Autodesk Inventor part; units mm, degrees
ref_plane "YZ Plane" through (0, 0, 0) normal (1, 0, 0) x (0, 1, 0)
ref_plane "XZ Plane" through (0, 0, 0) normal (0, 1, 0) x (-1, 0, 0)
ref_plane "XY Plane" through (0, 0, 0) normal (0, 0, 1) x (1, 0, 0)
sketch "Эскиз1" plane through (0, 0, 0) normal (0, 1, 0) x (-1, 0, 0)
  arc A0 (-8.6049, 20.7741) -> (-8.0517, 15.4673) centre (8.9595, 19.9228) ccw
  arc A1 (-8.0517, 15.4673) -> (-9.3692, 14.7066) centre (0, 0) ccw
  arc A2 (-9.3692, 14.7066) -> (-13.6885, 17.8391) centre (-21.7334, 2.2022) ccw
  arc A3 (-13.6885, 17.8391) -> (-15.1912, 16.5782) centre (0, 0) ccw
  arc A4 (-15.1912, 16.5782) -> (-12.8563, 11.7806) centre (1.6052, 21.7856) ccw
  arc A5 (-12.8563, 11.7806) -> (-13.8341, 10.6153) centre (0, 0) ccw
  arc A6 (-13.8341, 10.6153) -> (-18.9643, 12.0816) centre (-21.1759, -5.3638) ccw
  arc A7 (-18.9643, 12.0816) -> (-19.9451, 10.3828) centre (0, 0) ccw
  arc A8 (-19.9451, 10.3828) -> (-16.1101, 6.673) centre (-5.9427, 21.0208) ccw
  arc A9 (-16.1101, 6.673) -> (-16.6304, 5.2436) centre (0, 0) ccw
  arc A10 (-16.6304, 5.2436) -> (-21.9528, 4.8668) centre (-18.0643, -12.2829) ccw
  arc A11 (-21.9528, 4.8668) -> (-22.2934, 2.935) centre (0, 0) ccw
  arc A12 (-22.2934, 2.935) -> (-17.4209, 0.7606) centre (-12.7739, 17.7205) ccw
  arc A13 (-17.4209, 0.7606) -> (-17.4209, -0.7606) centre (0, 0) ccw
  arc A14 (-17.4209, -0.7606) -> (-22.2934, -2.935) centre (-12.7739, -17.7205) ccw
  arc A15 (-22.2934, -2.935) -> (-21.9528, -4.8668) centre (0, 0) ccw
  arc A16 (-21.9528, -4.8668) -> (-16.6304, -5.2436) centre (-18.0643, 12.2829) ccw
  arc A17 (-16.6304, -5.2436) -> (-16.1101, -6.673) centre (0, 0) ccw
  arc A18 (-16.1101, -6.673) -> (-19.9451, -10.3828) centre (-5.9427, -21.0208) ccw
  arc A19 (-19.9451, -10.3828) -> (-18.9643, -12.0816) centre (0, 0) ccw
  arc A20 (-18.9643, -12.0816) -> (-13.8341, -10.6153) centre (-21.1759, 5.3638) ccw
  arc A21 (-13.8341, -10.6153) -> (-12.8563, -11.7806) centre (0, 0) ccw
  arc A22 (-12.8563, -11.7806) -> (-15.1912, -16.5782) centre (1.6052, -21.7856) ccw
  arc A23 (-15.1912, -16.5782) -> (-13.6885, -17.8391) centre (0, 0) ccw
  arc A24 (-13.6885, -17.8391) -> (-9.3692, -14.7066) centre (-21.7334, -2.2022) ccw
  arc A25 (-9.3692, -14.7066) -> (-8.0517, -15.4673) centre (0, 0) ccw
  arc A26 (-8.0517, -15.4673) -> (-8.6049, -20.7741) centre (8.9595, -19.9228) ccw
  arc A27 (-8.6049, -20.7741) -> (-6.7616, -21.445) centre (0, 0) ccw
  arc A28 (-6.7616, -21.445) -> (-3.7742, -17.0242) centre (-19.6695, -9.5027) ccw
  arc A29 (-3.7742, -17.0242) -> (-2.2761, -17.2883) centre (0, 0) ccw
  arc A30 (-2.2761, -17.2883) -> (-0.9808, -22.4644) centre (15.2332, -15.6569) ccw
  arc A31 (-0.9808, -22.4644) -> (0.9808, -22.4644) centre (0, 0) ccw
  arc A32 (0.9808, -22.4644) -> (2.2761, -17.2883) centre (-15.2332, -15.6569) ccw
  arc A33 (2.2761, -17.2883) -> (3.7742, -17.0242) centre (0, 0) ccw
  arc A34 (3.7742, -17.0242) -> (6.7616, -21.445) centre (19.6695, -9.5027) ccw
  arc A35 (6.7616, -21.445) -> (8.6049, -20.7741) centre (0, 0) ccw
  arc A36 (8.6049, -20.7741) -> (8.0517, -15.4673) centre (-8.9595, -19.9228) ccw
  arc A37 (8.0517, -15.4673) -> (9.3692, -14.7066) centre (0, 0) ccw
  arc A38 (9.3692, -14.7066) -> (13.6885, -17.8391) centre (21.7334, -2.2022) ccw
  arc A39 (13.6885, -17.8391) -> (15.1912, -16.5782) centre (0, 0) ccw
  arc A40 (15.1912, -16.5782) -> (12.8563, -11.7806) centre (-1.6052, -21.7856) ccw
  arc A41 (12.8563, -11.7806) -> (13.8341, -10.6153) centre (0, 0) ccw
  arc A42 (13.8341, -10.6153) -> (18.9643, -12.0816) centre (21.1759, 5.3638) ccw
  arc A43 (18.9643, -12.0816) -> (19.9451, -10.3828) centre (0, 0) ccw
  arc A44 (19.9451, -10.3828) -> (16.1101, -6.673) centre (5.9427, -21.0208) ccw
  arc A45 (16.1101, -6.673) -> (16.6304, -5.2436) centre (0, 0) ccw
  arc A46 (16.6304, -5.2436) -> (21.9528, -4.8668) centre (18.0643, 12.2829) ccw
  arc A47 (21.9528, -4.8668) -> (22.2934, -2.935) centre (0, 0) ccw
  arc A48 (22.2934, -2.935) -> (17.4209, -0.7606) centre (12.7739, -17.7205) ccw
  arc A49 (17.4209, -0.7606) -> (17.4209, 0.7606) centre (0, 0) ccw
  arc A50 (17.4209, 0.7606) -> (22.2934, 2.935) centre (12.7739, 17.7205) ccw
  arc A51 (22.2934, 2.935) -> (21.9528, 4.8668) centre (0, 0) ccw
  arc A52 (21.9528, 4.8668) -> (16.6304, 5.2436) centre (18.0643, -12.2829) ccw
  arc A53 (16.6304, 5.2436) -> (16.1101, 6.673) centre (0, 0) ccw
  arc A54 (16.1101, 6.673) -> (19.9451, 10.3828) centre (5.9427, 21.0208) ccw
  arc A55 (19.9451, 10.3828) -> (18.9643, 12.0816) centre (0, 0) ccw
  arc A56 (18.9643, 12.0816) -> (13.8341, 10.6153) centre (21.1759, -5.3638) ccw
  arc A57 (13.8341, 10.6153) -> (12.8563, 11.7806) centre (0, 0) ccw
  arc A58 (12.8563, 11.7806) -> (15.1912, 16.5782) centre (-1.6052, 21.7856) ccw
  arc A59 (15.1912, 16.5782) -> (13.6885, 17.8391) centre (0, 0) ccw
  arc A60 (13.6885, 17.8391) -> (9.3692, 14.7066) centre (21.7334, 2.2022) ccw
  arc A61 (9.3692, 14.7066) -> (8.0517, 15.4673) centre (0, 0) ccw
  arc A62 (8.0517, 15.4673) -> (8.6049, 20.7741) centre (-8.9595, 19.9228) ccw
  arc A63 (8.6049, 20.7741) -> (6.7616, 21.445) centre (0, 0) ccw
  arc A64 (6.7616, 21.445) -> (3.7742, 17.0242) centre (19.6695, 9.5027) ccw
  arc A65 (3.7742, 17.0242) -> (2.2761, 17.2883) centre (0, 0) ccw
  arc A66 (2.2761, 17.2883) -> (0.9808, 22.4644) centre (-15.2332, 15.6569) ccw
  arc A67 (0.9808, 22.4644) -> (-0.9808, 22.4644) centre (0, 0) ccw
  arc A68 (-0.9808, 22.4644) -> (-2.2761, 17.2883) centre (15.2332, 15.6569) ccw
  arc A69 (-2.2761, 17.2883) -> (-3.7742, 17.0242) centre (0, 0) ccw
  arc A70 (-3.7742, 17.0242) -> (-6.7616, 21.445) centre (-19.6695, 9.5027) ccw
  arc A71 (-6.7616, 21.445) -> (-8.6049, 20.7741) centre (0, 0) ccw
  arc A72 (-5.2271, 12.6194) -> (-4.9205, 9.4522) centre (5.1709, 12.0276) ccw
  arc A73 (-4.9205, 9.4522) -> (-5.7256, 8.9874) centre (0, 0) ccw
  arc A74 (-5.7256, 8.9874) -> (-8.3151, 10.8365) centre (-13.0016, 1.5357) ccw
  arc A75 (-8.3151, 10.8365) -> (-9.228, 10.0706) centre (0, 0) ccw
  arc A76 (-9.228, 10.0706) -> (-7.8566, 7.1993) centre (0.7454, 13.0708) ccw
  arc A77 (-7.8566, 7.1993) -> (-8.4542, 6.4871) centre (0, 0) ccw
  arc A78 (-8.4542, 6.4871) -> (-11.52, 7.339) centre (-12.7428, -3.0038) ccw
  arc A79 (-11.52, 7.339) -> (-12.1158, 6.3071) centre (0, 0) ccw
  arc A80 (-12.1158, 6.3071) -> (-9.8451, 4.078) centre (-3.77, 12.5374) ccw
  arc A81 (-9.8451, 4.078) -> (-10.163, 3.2044) centre (0, 0) ccw
  arc A82 (-10.163, 3.2044) -> (-13.3353, 2.9564) centre (-10.9469, -7.1809) ccw
  arc A83 (-13.3353, 2.9564) -> (-13.5423, 1.7829) centre (0, 0) ccw
  arc A84 (-13.5423, 1.7829) -> (-10.6461, 0.4648) centre (-7.8307, 10.4919) ccw
  arc A85 (-10.6461, 0.4648) -> (-10.6461, -0.4648) centre (0, 0) ccw
  arc A86 (-10.6461, -0.4648) -> (-13.5423, -1.7829) centre (-7.8307, -10.4919) ccw
  arc A87 (-13.5423, -1.7829) -> (-13.3353, -2.9564) centre (0, 0) ccw
  arc A88 (-13.3353, -2.9564) -> (-10.163, -3.2044) centre (-10.9469, 7.1809) ccw
  arc A89 (-10.163, -3.2044) -> (-9.8451, -4.078) centre (0, 0) ccw
  arc A90 (-9.8451, -4.078) -> (-12.1158, -6.3071) centre (-3.77, -12.5374) ccw
  arc A91 (-12.1158, -6.3071) -> (-11.52, -7.339) centre (0, 0) ccw
  arc A92 (-11.52, -7.339) -> (-8.4542, -6.4871) centre (-12.7428, 3.0038) ccw
  arc A93 (-8.4542, -6.4871) -> (-7.8566, -7.1993) centre (0, 0) ccw
  arc A94 (-7.8566, -7.1993) -> (-9.228, -10.0706) centre (0.7454, -13.0708) ccw
  arc A95 (-9.228, -10.0706) -> (-8.3151, -10.8365) centre (0, 0) ccw
  arc A96 (-8.3151, -10.8365) -> (-5.7256, -8.9874) centre (-13.0016, -1.5357) ccw
  arc A97 (-5.7256, -8.9874) -> (-4.9205, -9.4522) centre (0, 0) ccw
  arc A98 (-4.9205, -9.4522) -> (-5.2271, -12.6194) centre (5.1709, -12.0276) ccw
  arc A99 (-5.2271, -12.6194) -> (-4.1074, -13.0269) centre (0, 0) ccw
  arc A100 (-4.1074, -13.0269) -> (-2.3064, -10.4037) centre (-11.6923, -5.8899) ccw
  arc A101 (-2.3064, -10.4037) -> (-1.3909, -10.5651) centre (0, 0) ccw
  arc A102 (-1.3909, -10.5651) -> (-0.5958, -13.6461) centre (8.9727, -9.5337) ccw
  arc A103 (-0.5958, -13.6461) -> (0.5958, -13.6461) centre (0, 0) ccw
  arc A104 (0.5958, -13.6461) -> (1.3909, -10.5651) centre (-8.9727, -9.5337) ccw
  arc A105 (1.3909, -10.5651) -> (2.3064, -10.4037) centre (0, 0) ccw
  arc A106 (2.3064, -10.4037) -> (4.1074, -13.0269) centre (11.6923, -5.8899) ccw
  arc A107 (4.1074, -13.0269) -> (5.2271, -12.6194) centre (0, 0) ccw
  arc A108 (5.2271, -12.6194) -> (4.9205, -9.4522) centre (-5.1709, -12.0276) ccw
  arc A109 (4.9205, -9.4522) -> (5.7256, -8.9874) centre (0, 0) ccw
  arc A110 (5.7256, -8.9874) -> (8.3151, -10.8365) centre (13.0016, -1.5357) ccw
  arc A111 (8.3151, -10.8365) -> (9.228, -10.0706) centre (0, 0) ccw
  arc A112 (9.228, -10.0706) -> (7.8566, -7.1993) centre (-0.7454, -13.0708) ccw
  arc A113 (7.8566, -7.1993) -> (8.4542, -6.4871) centre (0, 0) ccw
  arc A114 (8.4542, -6.4871) -> (11.52, -7.339) centre (12.7428, 3.0038) ccw
  arc A115 (11.52, -7.339) -> (12.1158, -6.3071) centre (0, 0) ccw
  arc A116 (12.1158, -6.3071) -> (9.8451, -4.078) centre (3.77, -12.5374) ccw
  arc A117 (9.8451, -4.078) -> (10.163, -3.2044) centre (0, 0) ccw
  arc A118 (10.163, -3.2044) -> (13.3353, -2.9564) centre (10.9469, 7.1809) ccw
  arc A119 (13.3353, -2.9564) -> (13.5423, -1.7829) centre (0, 0) ccw
  arc A120 (13.5423, -1.7829) -> (10.6461, -0.4648) centre (7.8307, -10.4919) ccw
  arc A121 (10.6461, -0.4648) -> (10.6461, 0.4648) centre (0, 0) ccw
  arc A122 (10.6461, 0.4648) -> (13.5423, 1.7829) centre (7.8307, 10.4919) ccw
  arc A123 (13.5423, 1.7829) -> (13.3353, 2.9564) centre (0, 0) ccw
  arc A124 (13.3353, 2.9564) -> (10.163, 3.2044) centre (10.9469, -7.1809) ccw
  arc A125 (10.163, 3.2044) -> (9.8451, 4.078) centre (0, 0) ccw
  arc A126 (9.8451, 4.078) -> (12.1158, 6.3071) centre (3.77, 12.5374) ccw
  arc A127 (12.1158, 6.3071) -> (11.52, 7.339) centre (0, 0) ccw
  arc A128 (11.52, 7.339) -> (8.4542, 6.4871) centre (12.7428, -3.0038) ccw
  arc A129 (8.4542, 6.4871) -> (7.8566, 7.1993) centre (0, 0) ccw
  arc A130 (7.8566, 7.1993) -> (9.228, 10.0706) centre (-0.7454, 13.0708) ccw
  arc A131 (9.228, 10.0706) -> (8.3151, 10.8365) centre (0, 0) ccw
  arc A132 (8.3151, 10.8365) -> (5.7256, 8.9874) centre (13.0016, 1.5357) ccw
  arc A133 (5.7256, 8.9874) -> (4.9205, 9.4522) centre (0, 0) ccw
  arc A134 (4.9205, 9.4522) -> (5.2271, 12.6194) centre (-5.1709, 12.0276) ccw
  arc A135 (5.2271, 12.6194) -> (4.1074, 13.0269) centre (0, 0) ccw
  arc A136 (4.1074, 13.0269) -> (2.3064, 10.4037) centre (11.6923, 5.8899) ccw
  arc A137 (2.3064, 10.4037) -> (1.3909, 10.5651) centre (0, 0) ccw
  arc A138 (1.3909, 10.5651) -> (0.5958, 13.6461) centre (-8.9727, 9.5337) ccw
  arc A139 (0.5958, 13.6461) -> (-0.5958, 13.6461) centre (0, 0) ccw
  arc A140 (-0.5958, 13.6461) -> (-1.3909, 10.5651) centre (8.9727, 9.5337) ccw
  arc A141 (-1.3909, 10.5651) -> (-2.3064, 10.4037) centre (0, 0) ccw
  arc A142 (-2.3064, 10.4037) -> (-4.1074, 13.0269) centre (-11.6923, 5.8899) ccw
  arc A143 (-4.1074, 13.0269) -> (-5.2271, 12.6194) centre (0, 0) ccw
extrude "Выдавливание1" add sketch "Эскиз1" along normal blind 5 contours A143 A142 A141 A140 A139 A138 A137 A136 A135 A134 A133 A132 A131 A130 A129 A128 A127 A126 A125 A124 A123 A122 A121 A120 A119 A118 A117 A116 A115 A114 A113 A112 A111 A110 A109 A108 A107 A106 A105 A104 A103 A102 A101 A100 A99 A98 A97 A96 A95 A94 A93 A92 A91 A90 A89 A88 A87 A86 A85 A84 A83 A82 A81 A80 A79 A78 A77 A76 A75 A74 A73 A72
sketch "Эскиз2" plane through (0, 5, 0) normal (0, 1, 0) x (1, 0, 0)
  arc A0 (14.2029, 0.3107) -> (13.9664, 4.3996) centre (13.4768, 2.32) ccw
  line L0 (13.9664, 4.3996) -> (5.393, 4.3996)
  line L1 (5.393, 4.3996) -> (6.8323, 12.4554)
  arc A1 (6.8323, 12.4554) -> (3.173, 14.2951) centre (4.7292, 12.8312) ccw
  line L2 (3.173, 14.2951) -> (-1.1137, 6.8702)
  line L3 (-1.1137, 6.8702) -> (-7.3706, 12.1447)
  arc A2 (-7.3706, 12.1447) -> (-10.7934, 9.8955) centre (-8.7476, 10.5112) ccw
  line L4 (-10.7934, 9.8955) -> (-6.5067, 2.4706)
  line L5 (-6.5067, 2.4706) -> (-14.2029, -0.3107)
  arc A3 (-14.2029, -0.3107) -> (-13.9664, -4.3996) centre (-13.4768, -2.32) ccw
  line L6 (-13.9664, -4.3996) -> (-5.393, -4.3996)
  line L7 (-5.393, -4.3996) -> (-6.8323, -12.4554)
  arc A4 (-6.8323, -12.4554) -> (-3.173, -14.2951) centre (-4.7292, -12.8312) ccw
  line L8 (-3.173, -14.2951) -> (1.1137, -6.8702)
  line L9 (1.1137, -6.8702) -> (7.3706, -12.1447)
  arc A5 (7.3706, -12.1447) -> (10.7934, -9.8955) centre (8.7476, -10.5112) ccw
  line L10 (10.7934, -9.8955) -> (6.5067, -2.4706)
  line L11 (6.5067, -2.4706) -> (14.2029, 0.3107)
  circle A6 centre (7.5637, 1.3021) radius 1
  circle A7 centre (13.4768, 2.32) radius 1
  circle A8 centre (6.8286, -8.2053) radius 1
  circle A9 centre (-2.6542, -7.2014) radius 1
  circle A10 centre (-4.7292, -12.8312) radius 1
  circle A11 centre (-10.5203, -1.8111) radius 1
  circle A12 centre (-4.9095, 5.8993) radius 1
  circle A13 centre (-8.7476, 10.5112) radius 1
  circle A14 centre (3.6917, 10.0163) radius 1
  circle A15 centre (0, 0) radius 4.75
  circle A16 centre (4.7292, 12.8312) radius 1
  circle A17 centre (2.6542, 7.2014) radius 1
  circle A18 centre (-6.8286, 8.2053) radius 1
  circle A19 centre (-13.4768, -2.32) radius 1
  circle A20 centre (-7.5637, -1.3021) radius 1
  circle A21 centre (-3.6917, -10.0163) radius 1
  circle A22 centre (8.7476, -10.5112) radius 1
  circle A23 centre (4.9095, -5.8993) radius 1
  circle A24 centre (10.5203, 1.8111) radius 1
  circle A25 centre (0, 0) radius 1.875
extrude "Выдавливание2" cut sketch "Эскиз2" against normal blind 10 contours A6 | A9 | A12 | A15 | A17 | A20 | A23 | A25
properties part number "000.303 - Шестерня привода"
Work out the finished part from the listing and answer in its coordinate system (mm). A direction names the side the tool comes from. Round coordinates to 2 decimals unless told otherwise and drop trailing zeros. Loops run counter-clockwise (first coordinate to the right, second up) from the corner with the lowest first, then second, coordinate; pieces in that order, holes last. Notation, with made-up numbers: (58.25, 56) - (70.25, 56) arc R16 ccw to (70.25, 77) - close; hole circle Ø9 at (-18, -9.75). An arc over 180 degrees is marked (long way). Use one line per item in the form item = value. Start each with the question number.
(1) Which of the six approach directions +Z, -Z, +X, -X, +Y, -Y give full straight-line access (tool end or side, diameter ignored) to faces 1 (the face through (-1.12, 2.46, -12.11)), 2 (the face through (1.857, 2.465, 10.493)), 3 (the face through (11.736, 2.465, -3.204)), 4 (the face through (12.165, 2.465, -1.022)), 5 (the face through (-12.165, 2.465, 1.022))?
(2) Find section A-A on x = 0. Determine the outline of the cut face in (y, z).
(3) Flat-ended cylindrical pins translate along their axes: P1, Ø1.5, axis at y = 0.5, z = -10.5, coming from the +X side; P2, Ø1, axis at x = 4.5, y = 4.5, coming from the +Z side; P3, Ø1.5, axis at x = -8, y = 1, coming from the -Z side. Find the tip coordinate at first contact, or state that the pin passes through.
(4) Find section B-B on z = -11.5. Determine the outline of the cut face in (x, y), and give its area (3 significant figures).
(5) Consider line 1 (Z direction, x = 11.5, y = 4); line 2 (X direction, y = 1.7, z = -11.5); line 3 (Z direction, x = -4, y = 3.65) (3 decimals). Determine where each line is inside the solid, lowest interval first.
(6) Find section C-C on y = 0.4. Give the number of separate pieces and of enclosed holes in the cut face, and give its area (3 significant figures).
(7) Determine the mould class of faces 6 (the face through (-11.8, 2.5, -3.2)), 7 (the face through (2.524, 2.535, -8.193)), 8 (the face through (8.786, 2.465, 10.458)), 9 (the face through (-4.68, 2.465, -12.832)) for opening direction Z: +Z half, -Z half, draft (parallel to the pull), parting line (faces both ways), or undercut.
Answer list:
q1.face_1 = -Z, +Y, -Y
q1.face_2 = +Z, +Y, -Y
q1.face_3 = +Y, -Y
q1.face_4 = +X, +Y, -Y
q1.face_5 = -X, +Y, -Y
q2.outline = (0, -13.66) - (5, -13.66) - (5, -4.75) - (0, -4.75) - close; (0, 4.75) - (5, 4.75) - (5, 13.66) - (0, 13.66) - close
q3.P1 = 9.23
q3.P2 = 13.03
q3.P3 = -10.84
q4.outline = (-5.23, 0) - (-2.92, 0) - (-2.92, 5) - (-5.23, 5) - close; (-1.25, 0) - (1.25, 0) - (1.25, 5) - (-1.25, 5) - close; (2.92, 0) - (5.23, 0) - (5.23, 5) - (2.92, 5) - close
q4.area = 35.7 mm^2
q5.line_1 = -7.34 to -5.56, -3.22 to -0.74, 0.74 to 3.22, 5.56 to 7.34
q5.line_2 = -5.23 to -2.92, -1.25 to 1.25, 2.92 to 5.23
q5.line_3 = -12.911 to -6.315, -5.484 to -2.562, 2.562 to 12.911
q6.separate_pieces = 1
q6.enclosed_holes = 7
q6.area = 384 mm^2
q7.face_6 = undercut
q7.face_7 = undercut
q7.face_8 = +Z half
q7.face_9 = -Z half
